CAD build for the part. Positions are in the model's coordinates, mm. Face numbers are marked on the shaded views. A direction names the side the tool comes from. Coordinates: 2 decimals unless noted, no trailing zeros. Write each loop counter-clockwise with the first axis right and the second up, starting at its lowest first coordinate (ties: lowest second). Pieces come first, ordered by that corner, then holes.
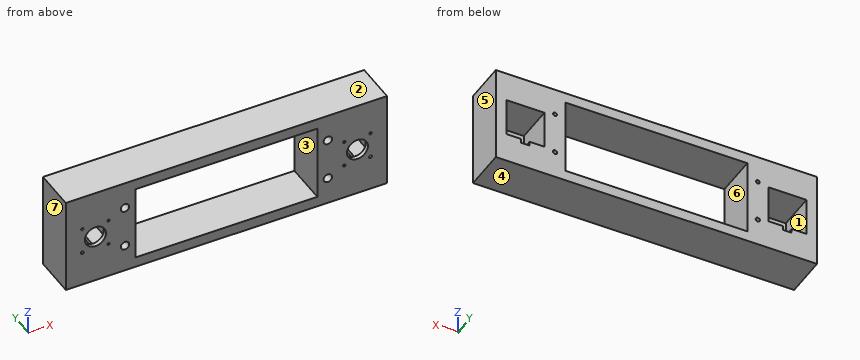
Autodesk Inventor part; units mm, degrees
ref_plane "YZ Plane" through (0, 0, 0) normal (1, 0, 0) x (0, 1, 0)
ref_plane "XZ Plane" through (0, 0, 0) normal (0, 1, 0) x (-1, 0, 0)
ref_plane "XY Plane" through (0, 0, 0) normal (0, 0, 1) x (1, 0, 0)
sketch "Sketch1" plane through (0, 0, 0) normal (0, 1, 0) x (-1, 0, 0)
  line L0 (190, -57.5) -> (-190, -57.5)
  line L1 (-190, -57.5) -> (-190, 57.5)
  line L2 (-190, 57.5) -> (190, 57.5)
  line L3 (190, 57.5) -> (190, -57.5)
  line L4 (0, -57.5) -> (0, 57.5) construction
  line L5 (190, 0) -> (-190, 0) construction
  point P0 (0, 0)
  point P1 (0, 0)
  dimension "d0" = 380
  dimension "d1" = 115
extrude "Extrusion1" add sketch "Sketch1" along normal blind 50
sketch "Sketch2" plane through (0, 50, 0) normal (0, 1, 0) x (1, 0, 0)
  line L0 (-177.5, 22.5) -> (-132.5, 22.5)
  line L1 (-132.5, 22.5) -> (-132.5, -22.5)
  line L2 (-132.5, -22.5) -> (-177.5, -22.5)
  line L3 (-177.5, -22.5) -> (-177.5, 22.5)
  line L4 (190, 57.5) -> (-190, 57.5) construction
  line L5 (0, 57.5) -> (0, -57.5) construction
  line L6 (-190, -57.5) -> (190, -57.5) construction
  line L7 (-190, 57.5) -> (-190, -57.5) construction
  line L8 (-190, 0) -> (190, 0) construction
  line L9 (190, -57.5) -> (190, 57.5) construction
  line L10 (-177.5, 0) -> (-132.5, 0) construction
  line L11 (-155, 22.5) -> (-155, -22.5) construction
  line L12 (177.5, 22.5) -> (132.5, 22.5)
  line L13 (132.5, 22.5) -> (132.5, -22.5)
  line L14 (132.5, -22.5) -> (177.5, -22.5)
  line L15 (177.5, -22.5) -> (177.5, 22.5)
  point P0 (0, 0)
  dimension "d4" = 45
  dimension "d5" = 45
  dimension "d6" = 310
extrude "Extrusion2" cut sketch "Sketch2" against normal blind 45
sketch "Sketch3" plane through (0, 50, 0) normal (0, 1, 0) x (1, 0, 0)
  line L0 (190, 57.5) -> (-190, 57.5) construction
  line L1 (0, 57.5) -> (0, -57.5) construction
  line L2 (-190, -57.5) -> (190, -57.5) construction
  line L3 (-132.5, 22.5) -> (-132.5, -22.5) construction
  line L4 (-132.5, 0) -> (132.5, 0) construction
  line L5 (132.5, -22.5) -> (132.5, 22.5) construction
  line L6 (-120, 25) -> (-120, -25) construction
  circle A0 centre (-120, 25) radius 2.5
  circle A1 centre (-120, -25) radius 2.25
  circle A2 centre (120, 25) radius 2.5
  circle A3 centre (120, -25) radius 2.25
  point P0 (0, 0)
  dimension "d15" = 50
  dimension "d16" = 5
  dimension "d17" = 4.5
  dimension "d18" = 50
  dimension "d19" = 240
extrude "Extrusion3" cut sketch "Sketch3" against normal up to next
sketch "Sketch4" plane through (0, 50, 0) normal (0, 1, 0) x (1, 0, 0)
  line L0 (107.5, -45) -> (-107.5, -45)
  line L1 (-107.5, -45) -> (-107.5, 45)
  line L2 (-107.5, 45) -> (107.5, 45)
  line L3 (107.5, 45) -> (107.5, -45)
  line L4 (0, -45) -> (0, 45) construction
  line L5 (107.5, 0) -> (-107.5, 0) construction
  circle A0 centre (120, -25) radius 2.25
  point P0 (0, 0)
  point P1 (0, 0)
  dimension "d23" = 90
  dimension "d29" = 12.5
extrude "Extrusion4" cut sketch "Sketch4" against normal up to next contours L0 L1 L2 L3
sketch "Sketch5" plane through (0, 5, 0) normal (0, 1, 0) x (1, 0, 0)
  line L0 (-190, -57.5) -> (190, -57.5) construction
  line L1 (0, -57.5) -> (0, 57.5) construction
  line L2 (190, 57.5) -> (-190, 57.5) construction
  line L3 (132.5, -22.5) -> (132.5, 22.5) construction
  line L4 (177.5, -22.5) -> (132.5, -22.5) construction
  line L5 (177.5, 22.5) -> (177.5, -22.5) construction
  line L6 (132.5, 22.5) -> (177.5, 22.5) construction
  line L7 (177.5, -22.5) -> (132.5, -22.5) construction
  line L8 (155, -22.5) -> (155, 22.5) construction
  line L9 (132.5, 22.5) -> (177.5, 22.5) construction
  line L10 (177.5, 22.5) -> (177.5, -22.5) construction
  line L11 (177.5, 0) -> (132.5, 0) construction
  line L12 (132.5, -22.5) -> (132.5, 22.5) construction
  circle A0 centre (155, 0) radius 12.5
  circle A1 centre (-155, 0) radius 12.5
  point P0 (0, 0)
  dimension "d26" = 25
extrude "Extrusion5" cut sketch "Sketch5" against normal up to next
sketch "Sketch6" plane through (0, 5, 0) normal (0, 1, 0) x (1, 0, 0)
  line L0 (190, 57.5) -> (-190, 57.5) construction
  line L1 (0, 57.5) -> (0, -57.5) construction
  line L2 (190, -57.5) -> (-190, -57.5) construction
  line L3 (-170.5, 15.5) -> (-139.5, 15.5) construction
  line L4 (-139.5, 15.5) -> (-139.5, -15.5) construction
  line L5 (-139.5, -15.5) -> (-170.5, -15.5) construction
  line L6 (-170.5, -15.5) -> (-170.5, 15.5) construction
  line L7 (-177.5, 22.5) -> (-132.5, 22.5) construction
  line L8 (-132.5, -22.5) -> (-177.5, -22.5) construction
  line L9 (-155, 22.5) -> (-155, -22.5) construction
  line L10 (-177.5, -22.5) -> (-177.5, 22.5) construction
  line L11 (-177.5, 0) -> (-132.5, 0) construction
  line L12 (-132.5, 22.5) -> (-132.5, -22.5) construction
  line L13 (-170.5, 0) -> (-139.5, 0) construction
  line L14 (-155, -15.5) -> (-155, 15.5) construction
  circle A0 centre (-170.5, 15.5) radius 1.75
  circle A1 centre (-139.5, 15.5) radius 1.5
  circle A2 centre (-170.5, -15.5) radius 1.5
  circle A3 centre (-139.5, -15.5) radius 1.5
  circle A4 centre (170.5, 15.5) radius 1.75
  circle A5 centre (139.5, 15.5) radius 1.5
  circle A6 centre (170.5, -15.5) radius 1.5
  circle A7 centre (139.5, -15.5) radius 1.5
  point P0 (0, 0)
  point P1 (-155, 0)
  dimension "d30" = 31
  dimension "d31" = 31
  dimension "d32" = 3.5
  dimension "d33" = 3
  dimension "d34" = 3
  dimension "d35" = 3
extrude "Extrusion6" cut sketch "Sketch6" against normal up to next
sketch "Sketch7" plane through (0, 50, 0) normal (0, 1, 0) x (1, 0, 0)
  line L0 (-190, 57.5) -> (190, 57.5) construction
  line L1 (0, 57.5) -> (0, -57.5) construction
  line L2 (190, -57.5) -> (-190, -57.5) construction
  line L3 (-177.5, 22.5) -> (-132.5, 22.5)
  line L4 (-160, 22.5) -> (-150, 22.5)
  line L5 (-150, 22.5) -> (-150, 27.5)
  line L6 (-150, 27.5) -> (-160, 27.5)
  line L7 (-160, 27.5) -> (-160, 22.5)
  line L8 (-155, 27.5) -> (-155, 22.5) construction
  line L9 (160, 22.5) -> (150, 22.5)
  line L10 (150, 22.5) -> (150, 27.5)
  line L11 (150, 27.5) -> (160, 27.5)
  line L12 (160, 27.5) -> (160, 22.5)
  point P0 (0, 0)
  dimension "d38" = 10
  dimension "d39" = 5
  dimension "d40" = 22.5
extrude "Extrusion7" cut sketch "Sketch7" against normal blind 45
sketch "Sketch8" plane through (0, 0, 0) normal (0, -1, 0) x (1, 0, 0)
  circle A0 centre (-120, 25) radius 2.25
  circle A1 centre (-120, 25) radius 5
  line L0 (-190, -57.5) -> (-190, 57.5) construction
  line L1 (-190, 0) -> (190, 0) construction
  line L2 (190, 57.5) -> (190, -57.5) construction
  line L3 (-190, -57.5) -> (190, -57.5) construction
  line L4 (0, -57.5) -> (0, 57.5) construction
  line L5 (190, 57.5) -> (-190, 57.5) construction
  circle A2 centre (-120, -25) radius 5
  circle A3 centre (120, 25) radius 5
  circle A4 centre (120, -25) radius 5
  point P0 (0, 0)
  dimension "d43" = 10
extrude "Extrusion8" cut sketch "Sketch8" against normal blind 40
properties part number "antennae_holder"
Item 1: Flat gauge pins, fed straight in: pin 1 Ø4 at (x, z) = (-139.5, 15.5) entering from +Y; pin 2 Ø3 at (x, z) = (-120, -25) entering from -Y. Where does each tip first touch, or does it go through?
Item 2: Two-plate mould, pull along X, no slides. Class the marked faces 4, 5, 6 and 7: +X half, -X half, draft (parallel to the pull), parting line (faces both ways), or undercut.
Item 3: Saw through at C-C, the plane z = -7. Write the cut outline in (x, y).
Item 4: Saw through at D-D, the plane x = -155. Write the cut outline in (y, z), and give its area (4 significant figures).
Item 5: Wall check: line 1 along X through (y, z) = (18.5, -13); line 2 along X through (y, z) = (40, -33); line 3 along X through (y, z) = (1.6, -15.5). Give the ranges that are in metal, low to high.
Item 6: Saw through at A-A, the plane x = -9. Write the cut outline in (y, z).
Item 7: Which spindle directions (+Z, -Z, +X, -X, +Y, -Y) get a long thin tool onto all of the face, cutting with end or side? Do the marked faces 1, 2 and 3. Say none if no direction does.
Item 8: Saw through at B-B, the plane y = 28. Write the cut outline in (x, z).
Working result:
1. pin 1: stops at y = 5
1. pin 2: passes through
2. face 4: draft
2. face 5: +X half
2. face 6: undercut
2. face 7: -X half
3. outline: (-190, 0) - (-165.36, 0) - (-165.36, 5) - (-177.5, 5) - (-177.5, 50) - (-190, 50) - close; (-144.64, 0) - (-107.5, 0) - (-107.5, 50) - (-132.5, 50) - (-132.5, 5) - (-144.64, 5) - close; (107.5, 0) - (144.64, 0) - (144.64, 5) - (132.5, 5) - (132.5, 50) - (107.5, 50) - close; (165.36, 0) - (190, 0) - (190, 50) - (177.5, 50) - (177.5, 5) - (165.36, 5) - close
4. outline: (0, -57.5) - (50, -57.5) - (50, -27.5) - (5, -27.5) - (5, -12.5) - (0, -12.5) - close; (0, 12.5) - (5, 12.5) - (5, 22.5) - (50, 22.5) - (50, 57.5) - (0, 57.5) - close
4. area: 3,375 mm2
5. line 1: x = -190 to -177.5, -132.5 to -107.5, 107.5 to 132.5, 177.5 to 190
5. line 2: x = -190 to -107.5, 107.5 to 190
5. line 3: x = -190 to -172.25, -168.75 to -141, -138 to -107.5, 107.5 to 138, 141 to 168.75, 172.25 to 190
6. outline: (0, -57.5) - (50, -57.5) - (50, -45) - (0, -45) - close; (0, 45) - (50, 45) - (50, 57.5) - (0, 57.5) - close
7. face 1: +Y
7. face 2: +Z, +X, -X, +Y, -Y
7. face 3: +Y, -Y
8. outline: (-190, -57.5) - (190, -57.5) - (190, 57.5) - (-190, 57.5) - close; hole (-177.5, -22.5) - (-160, -22.5) - (-160, -27.5) - (-150, -27.5) - (-150, -22.5) - (-132.5, -22.5) - (-132.5, 22.5) - (-177.5, 22.5) - close; hole circle Ø10 at (-120, -25); hole circle Ø10 at (-120, 25); hole (-107.5, -45) - (107.5, -45) - (107.5, 45) - (-107.5, 45) - close; hole circle Ø10 at (120, -25); hole circle Ø10 at (120, 25); hole (132.5, -22.5) - (150, -22.5) - (150, -27.5) - (160, -27.5) - (160, -22.5) - (177.5, -22.5) - (177.5, 22.5) - (132.5, 22.5) - close
